from build123d import *

# Parameters (mm, degrees)
SKETCH_W     = 15
SKETCH_H     = 41.5
PAD_DEPTH    = 3
SKETCH001_W  = 15
SKETCH001_H  = 3
PAD001_DEPTH = 15
SKETCH002_W  = 3.8
SKETCH002_H  = 10
POCKET_DEPTH = 3
FILLET_R     = 4
FILLET001_R  = 1
FILLET002_R  = 1


with BuildPart() as part:
    # Sketch → Pad (new body)
    with BuildSketch(Plane.XY):
        with Locations((7.5, 20.75)):
            Rectangle(SKETCH_W, SKETCH_H)
    extrude(amount=PAD_DEPTH)

    # Sketch001 (on Face6 of Pad) → Pad001 (join)
    with BuildSketch(Plane.XY.offset(3)):
        with Locations((7.5, 1.5)):
            Rectangle(SKETCH001_W, SKETCH001_H)
    extrude(amount=PAD001_DEPTH)

    # Sketch002 (on Face7 of Pad001) → Pocket (cut)
    with BuildSketch(Plane.XY.offset(3)):
        with Locations((7.5, 36.5)):
            Rectangle(SKETCH002_W, SKETCH002_H)
    extrude(amount=-POCKET_DEPTH, mode=Mode.SUBTRACT)

    # Fillet
    fillet_edges = [part.edges().sort_by_distance(p)[0] for p in [
        (0, 41.5, 1.5),
        (15, 41.5, 1.5),
    ]]
    fillet(fillet_edges, radius=FILLET_R)

    # Fillet001
    fillet001_edges = [part.edges().sort_by_distance(p)[0] for p in [
        (13.828427, 40.328427, 3),
        (13.828427, 40.328427, 0),
        (4.8, 41.5, 3),
        (4.8, 41.5, 0),
        (5.6, 41.5, 1.5),
        (5.6, 36.5, 0),
        (5.6, 36.5, 3),
        (9.4, 36.5, 3),
        (7.5, 31.5, 3),
        (9.4, 41.5, 1.5),
        (9.4, 36.5, 0),
        (7.5, 31.5, 0),
        (9.4, 31.5, 1.5),
        (5.6, 31.5, 1.5),
    ]]
    fillet(fillet001_edges, radius=FILLET001_R)

    # Fillet002
    fillet002_edges = [part.edges().sort_by_distance(p)[0] for p in [
        (7.5, 3, 18),
        (0, 1.5, 18),
        (7.5, 0, 18),
        (15, 1.5, 18),
        (0, 3, 10.5),
        (0, 0, 10.5),
        (15, 3, 10.5),
        (15, 0, 10.5),
    ]]
    fillet(fillet002_edges, radius=FILLET002_R)


solid = part.part
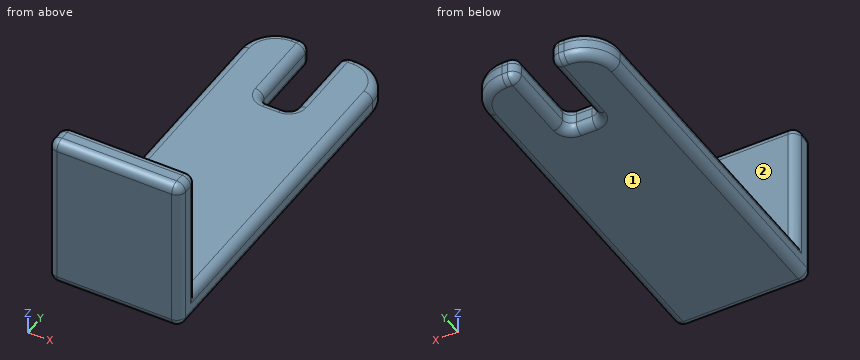
Input: part model. Units: mm. Frame: model coordinates. Face numbers are marked on the shaded views. A direction names the side the tool comes from. Round coordinates to 2 decimals unless told otherwise and drop trailing zeros. Order: outer loops, then holes, each group sorted by start corner. A loop starts at its lowest first (then second) coordinate and runs counter-clockwise, first axis right, second up. Notation, with made-up numbers: (-38.5, -20.75) - (-13.5, -20.75) arc R23 ccw to (-13.5, 6.25) - close; hole circle Ø6 at (17, 25.25). An arc over 180 degrees is marked (long way). Answer as a JSON object with one key per item and string values. Group by question number.
(1) Cut plane B-B (x = 8). Return loops of the section in (y, z).
(2) Cut plane C-C (y = 27). Return loops of the section in (x, z).
(3) Material intervals for probe 1 along Z at (x, y) = (3, 21); probe 2 along X at (y, z) = (34, 2.75), sorted ascending. Write a range as from..to.
(4) Pin query (flat end, axial travel): P1, Ø6.5, axis at x = 6.5, z = 7.5, coming from the +Y side; P2, Ø8, axis at x = 5.5, y = 30, coming from the +Z side; P3, Ø0.5, axis at x = 8, z = 1.5, coming from the +Y side. Return the tip coordinate at first contact, or that it passes through.
(5) Cut plane A-A (y = 34). Return loops of the section in (x, z), then the cut area to 3 significant figures.
(6) Reachability of the marked faces 1 and 2 from +Z, -Z, +X, -X, +Y, -Y: full face, straight path, thin tool, end or side. Return the list, or none.
Here are the results:
{
 "1": {"outline": "(0, 1) arc R1 ccw to (1, 0) - (30.5, 0) arc R1 ccw to (31.5, 1) - (31.5, 2) arc R1 ccw to (30.5, 3) - (3, 3) - (3, 17) arc R1 ccw to (2, 18) - (1, 18) arc R1 ccw to (0, 17) - close"},
 "2": {"outline": "(0, 1) arc R1 ccw to (1, 0) - (14, 0) arc R1 ccw to (15, 1) - (15, 2) arc R1 ccw to (14, 3) - (1, 3) arc R1 ccw to (0, 2) - close"},
 "3": {"probe 1": "z = 0..3", "probe 2": "x = 0.34..5.26, 9.74..14.66"},
 "4": {"P1": "stops at y = 3", "P2": "stops at z = 3", "P3": "stops at y = 31.5"},
 "5": {"outline": "(0, 1) arc R1 ccw to (1, 0) - (4.6, 0) arc R1 ccw to (5.6, 1) - (5.6, 2) arc R1 ccw to (4.6, 3) - (1, 3) arc R1 ccw to (0, 2) - close; (9.4, 1) arc R1 ccw to (10.4, 0) - (14, 0) arc R1 ccw to (15, 1) - (15, 2) arc R1 ccw to (14, 3) - (10.4, 3) arc R1 ccw to (9.4, 2) - close", "area": "31.9 mm^2"},
 "6": {"face 1": "-Z, +X, -X, +Y, -Y", "face 2": "+Z, +X, -X, +Y"}
}
